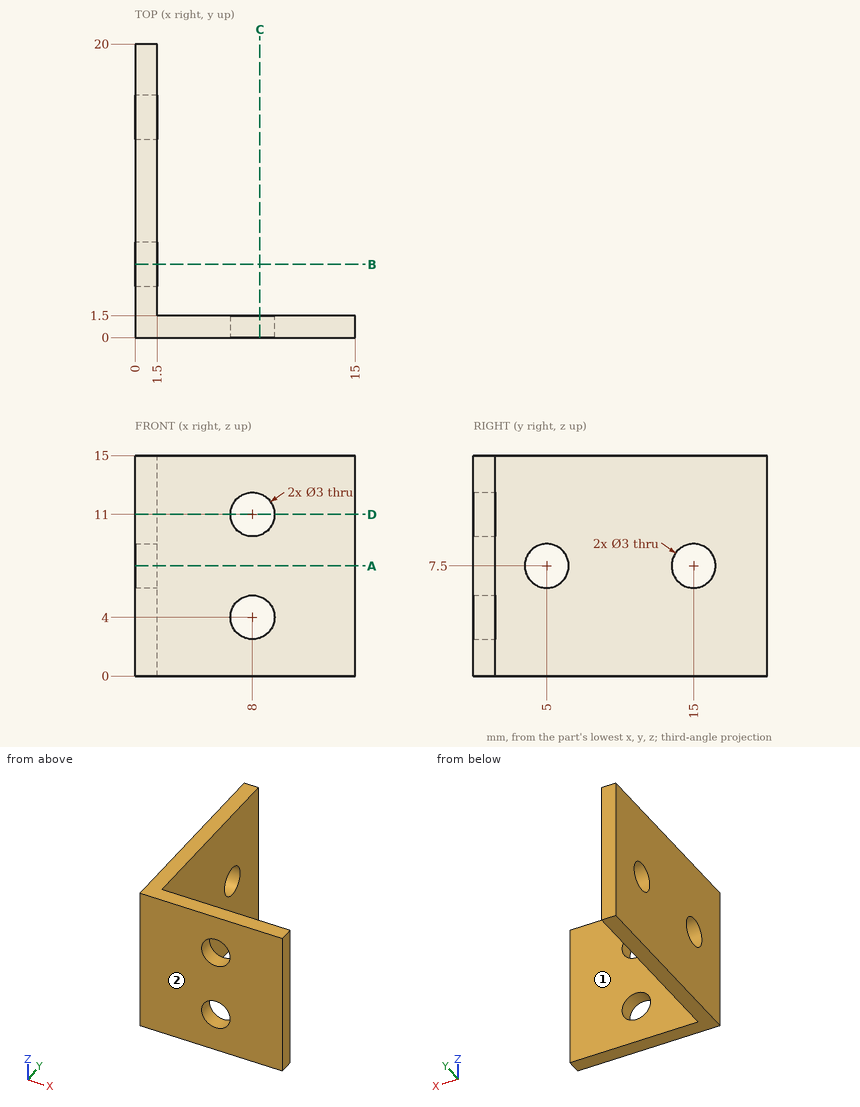
Study the drawing (mm; zero at the part's minimum x, y, z) and answer. A direction names the side the tool comes from. Give positions to 0.01 mm unless a question says otherwise; leave off trailing zeros. Write each loop counter-clockwise with the first axis right and the second up, starting at its lowest first coordinate (ties: lowest second). Pieces come first, ordered by that corner, then holes. Notation, with made-up numbers: M -22.5,4.25 L 33.5,4.25 A24 ccw 33.5,34.25 Z; hole C -14.75,-16 d9. An arc over 180 degrees is marked long. Put each result on its own line as item: value. Start each with the question number.
1. The part is cut by section B-B, the plane y = 5. Give the vertices of the cut face in (x, z), and give its area (3 significant figures).
2. Consider line 1 along Z through (x, y) = (8, 0.4); line 2 along Z through (x, y) = (0.85, 5); line 3 along X through (y, z) = (3.75, 1.5). Determine where each line is inside the solid, lowest interval first.
3. Each of these flat-tipped pins is pushed along its axis until it touches: pin 1 Ø2.5 at (x, z) = (8, 4) entering from +Y; pin 2 Ø4 at (y, z) = (15, 7.5) entering from +X. Where does it stop, or does it pass through?
4. Which of the six approach directions +Z, -Z, +X, -X, +Y, -Y give full straight-line access (tool end or side, diameter ignored) to the marked faces 1 and 2?
5. The part is cut by section A-A, the plane z = 7.5. Give the vertices of the cut face in (x, y).
6. The part is cut by section C-C, the plane x = 8.5. Give the vertices of the cut face in (y, z).
7. The part is cut by section D-D, the plane z = 11. Give the vertices of the cut face in (x, y).
Final values:
1. outline: M 0,0 L 1.5,0 L 1.5,6 L 0,6 Z; M 0,9 L 1.5,9 L 1.5,15 L 0,15 Z
1. area: 18.0 mm²
2. line 1: z = 0 to 2.5, 5.5 to 9.5, 12.5 to 15
2. line 2: z = 0 to 6, 9 to 15
2. line 3: x = 0 to 1.5
3. pin 1: passes through
3. pin 2: stops at x = 1.5
4. face 1: +Z, -Z, +X, +Y
4. face 2: +Z, -Z, +X, -X, -Y
5. outline: M 0,0 L 15,0 L 15,1.5 L 1.5,1.5 L 1.5,3.5 L 0,3.5 Z; M 0,6.5 L 1.5,6.5 L 1.5,13.5 L 0,13.5 Z; M 0,16.5 L 1.5,16.5 L 1.5,20 L 0,20 Z
6. outline: M 0,0 L 1.5,0 L 1.5,2.59 L 0,2.59 Z; M 0,5.41 L 1.5,5.41 L 1.5,9.59 L 0,9.59 Z; M 0,12.41 L 1.5,12.41 L 1.5,15 L 0,15 Z
7. outline: M 0,0 L 6.5,0 L 6.5,1.5 L 1.5,1.5 L 1.5,20 L 0,20 Z; M 9.5,0 L 15,0 L 15,1.5 L 9.5,1.5 Z
